```python
from build123d import *

# Parameters (mm, degrees)
P_IDAT_VYSUNUT_M1_DEPTH = 0.8


with BuildPart() as part:
    # Skica1 → Přidat vysunutím1 (new, symmetric)
    with BuildSketch(Plane(origin=(0, 0, 0), x_dir=(1, 0, 0), z_dir=(0, 1, 0))):
        with BuildLine():
            Line((21.590966819, 1.114633571), (21.584116759, -0.485351766))
            Line((21.584116759, -0.485351766), (29.204046923, -0.517975177))
            ThreePointArc((29.204046923, -0.517975177), (36.502348534, 2.047731055), (40.53322014, 8.650770428))
            Line((40.53322014, 8.650770428), (35.585436473, 7.930050796))
            Line((35.585436473, 7.930050796), (35.354806191, 9.513341569))
            Line((35.354806191, 9.513341569), (27.814383883, 8.41496485))
            Line((27.814383883, 8.41496485), (28.045014165, 6.831674076))
            Line((28.045014165, 6.831674076), (23.097230499, 6.110954444))
            Line((23.097230499, 6.110954444), (22.866600217, 7.694245217))
            Line((22.866600217, 7.694245217), (18.590994313, 1.127477433))
            Line((18.590994313, 1.127477433), (21.590966819, 1.114633571))
        make_face()
    extrude(amount=P_IDAT_VYSUNUT_M1_DEPTH, both=True)


solid = part.part
```
Verification items for the finished model (mm, model axes). A direction names the side the tool comes from. Coordinates: 2 decimals unless noted, no trailing zeros. Loops run counter-clockwise (first coordinate to the right, second up) from the corner with the lowest first, then second, coordinate; pieces in that order, holes last. Notation, with made-up numbers: (88.25, -31) - (95.25, -31) arc R8 cw to (95.25, -22) - close; hole circle Ø4 at (1, -33.5). An arc over 180 degrees is marked (long way). Answer as a JSON object with one key per item and string values.
(1) Cross-section at C-C, the plane x = 26.5. Record the boundary of the cut face in (y, z).
Response:
{"outline": "(-0.8, -6.61) - (0.8, -6.61) - (0.8, 0.51) - (-0.8, 0.51) - close"}
(2) Access from +Z, -Z, +X, -X, +Y, -Y to the whole of each face (thin tool, end or side, straight path). Record for faces 1 (the flat face through (22.984, 0.011, -6.892)), 2 (the flat face through (31.637, 0.011, -8.972)), 3 (the flat face through (27.93, 0.01, -7.63)).
Response:
{"face 1": "-Z, +Y, -Y", "face 2": "-Z, -X, +Y, -Y", "face 3": "+Y, -Y"}
(3) Cross-section at B-B, the plane y = 0.6. Record the boundary of the cut face in (x, z), then the cut area to 3 significant figures.
Response:
{"outline": "(18.59, -1.13) - (22.87, -7.69) - (23.1, -6.11) - (28.05, -6.83) - (27.81, -8.41) - (35.35, -9.51) - (35.59, -7.93) - (40.53, -8.65) arc R11.52 ccw to (29.2, 0.52) - (21.58, 0.49) - (21.59, -1.11) - close", "area": "142 mm²"}
(4) Cross-section at D-D, the plane z = -5.25. Record the boundary of the cut face in (x, y).
Response:
{"outline": "(21.28, -0.8) - (39.24, -0.8) - (39.24, 0.8) - (21.28, 0.8) - close"}
(5) Scan lines: line 1 along X through (y, z) = (-0.2, -5.75); line 2 along X through (y, z) = (0.25, -0.5); line 3 along X through (y, z) = (-0.5, -7.5). Record each from-to range of solid material in increasing order.
Response:
{"line 1": "x = 21.6 to 39.51", "line 2": "x = 21.59 to 33.99", "line 3": "x = 22.74 to 22.89, 27.95 to 40.23"}
(6) Cross-section at A-A, the plane z = -6.5. Record the boundary of the cut face in (x, y), then the cut area to 3 significant figures.
Response:
{"outline": "(22.09, -0.8) - (23.04, -0.8) - (23.04, 0.8) - (22.09, 0.8) - close; (25.77, -0.8) - (39.86, -0.8) - (39.86, 0.8) - (25.77, 0.8) - close", "area": "24.1 mm²"}
(7) Mould release check, pull along X, two halves, no side actions. Record for faces 4 (the flat face through (20.76, 0.01, -4.46)), 5 (the flat face through (35.47, 0.01, -8.71)), 6 (the flat face through (29, 0.8, -3)): pulls with the +X half, pulls with the -X half, needs draft (parallel to the pull), parting line crosses it, or undercut.
Response:
{"face 4": "pulls with the -X half", "face 5": "undercut", "face 6": "needs draft"}
